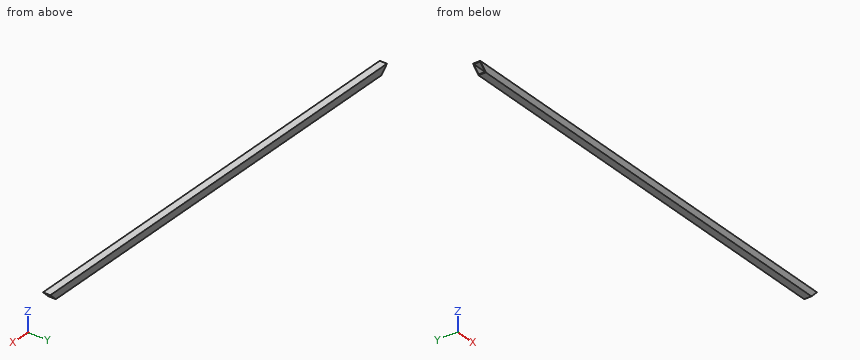
```python
from build123d import *

# Parameters (mm, degrees)
F0_W     = 25
F0_H     = 25
F1_DEPTH = 1524
F3_DEPTH = 12.5
F4_W     = 22
F4_H     = 22
F5_DEPTH = 1524.001


with BuildPart() as f1:
    # F0 (on Right) → F1 (new body)
    with BuildSketch(Plane.YZ):
        Rectangle(F0_W, F0_H)
    extrude(amount=F1_DEPTH)

    # F2 (on Front) → F3 (cut, symmetric)
    with BuildSketch(Plane.XZ):
        Polygon((35.352029, -22.745401), (0, 12.606628), (0, -26.686775), align=None)
        Polygon((1524, -22.745401), (1524, 12.5), (1494.63703, -16.86297), align=None)
    extrude(amount=F3_DEPTH, both=True, mode=Mode.SUBTRACT)

    # F4 (on Right) → F5 (cut, through all)
    with BuildSketch(Plane.YZ):
        Rectangle(F4_W, F4_H)
    extrude(amount=F5_DEPTH, mode=Mode.SUBTRACT)


solid = f1.part
```
Source: CAD feature listing. Evaluate the final solid. Frame: model axes, mm. Coordinates: 2 decimals unless noted, no trailing zeros. Write each loop counter-clockwise with the first axis right and the second up, starting at its lowest first coordinate (ties: lowest second). Pieces come first, ordered by that corner, then holes. Notation, with made-up numbers: (56, -18.75) - (110, -18.75) arc R17 ccw to (110, 12.25) - close; hole circle Ø5 at (-9, 38.25). An arc over 180 degrees is marked (long way). Answer as a JSON object with one key per item and string values.
Q1. Section query A-A, the plane y = -6.25. Output: boundary loops of the cut face in (x, z), plus the area to 3 significant figures.
Ans:
{"outline": "(0.11, 12.5) - (1.61, 11) - (1522.5, 11) - (1524, 12.5) - close; (23.61, -11) - (25.11, -12.5) - (1499, -12.5) - (1500.5, -11) - close", "area": "4,500 mm2"}
Q2. Material intervals for line 1 (Y direction, x = 854.5, z = 4.5); line 2 (X direction, y = -11.25, z = -3.25), sorted ascending. Write a range as [from, to].
Ans:
{"line 1": "y = [-12.5, -11], [11, 12.5]", "line 2": "x = [15.86, 1508.25]"}
Q3. Section query B-B, the plane z = -3. Output: boundary loops of the cut face in (x, y), plus the area to 3 significant figures.
Ans:
{"outline": "(15.61, -12.5) - (1508.5, -12.5) - (1508.5, -11) - (15.61, -11) - close; (15.61, 11) - (1508.5, 11) - (1508.5, 12.5) - (15.61, 12.5) - close", "area": "4,480 mm2"}
Q4. Section query C-C, the plane x = 1349. Output: boundary loops of the cut face in (y, z).
Ans:
{"outline": "(-12.5, -12.5) - (12.5, -12.5) - (12.5, 12.5) - (-12.5, 12.5) - close; hole (-11, -11) - (11, -11) - (11, 11) - (-11, 11) - close"}
Q5. First-contact query: pin 1 Ø10 at (y, z) = (9, 5) entering from +X. Flat tip, straight axial feed; report the tip coordinate or a pass-through.
Ans:
{"pin 1": "stops at x = 1521.08"}
